Source: CAD feature listing. Evaluate the final solid. Frame: model axes, mm. Coordinates: 2 decimals unless noted, no trailing zeros. Write each loop counter-clockwise with the first axis right and the second up, starting at its lowest first coordinate (ties: lowest second). Pieces come first, ordered by that corner, then holes. Notation, with made-up numbers: M 45,-8 L 77,-8 A32 ccw 77,22 Z; hole C 2,78 d1. An arc over 180 degrees is marked long. Write item = value, one per line. Start each with the question number.
1. Section query A-A (z = -1.8). Output: boundary loops of the cut face in (x, y).
2. Line query: line 1 along Y through (x, z) = (-149, -0.3); line 2 along X through (y, z) = (227, -1.55); line 3 along Y through (x, z) = (-171.5, -0.25). Output: solid intervals per line, ascending.
3. Pull-direction query (X, two-part tool) for faces 1 (the face through (-232.355, 188.231, -1.519)), 2 (the face through (-111.161, 214.644, -1.519)), 3 (the face through (-173, 205, -3)); classes: pulls with the +X half, pulls with the -X half, needs draft (parallel to the pull), parting line crosses it, or undercut.
4. Pin query (flat end, axial travel): pin 1 Ø1.5 at (x, z) = (-133, -2.5) entering from -Y. Return the tip coordinate at first contact, or that it passes through.
```python
from build123d import *

# Parameters (mm, degrees)
SKETCH_1_R      = 9
EXTRUDE_1_DEPTH = 3
FILLET_1_R      = 30
FILLET_2_R      = 0.15


with BuildPart() as part:
    # 草图1 → 凸台-拉伸1 (new body)
    with BuildSketch(Plane.XY):
        with Locations((-244.136401891, 191.197879466)):
            Circle(SKETCH_1_R)
        with Locations((-101.472478495, 222.230200701)):
            Circle(SKETCH_1_R)
        with BuildLine():
            Line((-100.516002841, 217.833024979), (-243.179926237, 186.800703745))
            ThreePointArc((-243.179926237, 186.800703745), (-248.533577612, 190.241403811), (-245.092877546, 195.595055187))
            Line((-245.092877546, 195.595055187), (-102.42895415, 226.627376422))
            ThreePointArc((-102.42895415, 226.627376422), (-97.075302774, 223.186676355), (-100.516002841, 217.833024979))
        make_face()
    extrude(amount=-EXTRUDE_1_DEPTH)

    # 圆角1
    fillet_1_edges = [part.edges().sort_by_distance(p)[0] for p in [
        (-108.132134599, 216.17636055, -1.5),
        (-235.563794478, 188.457368174, -1.5),
        (-237.476745787, 197.251719617, -1.5),
        (-110.045085908, 224.970711992, -1.5),
    ]]
    fillet(fillet_1_edges, radius=FILLET_1_R)

    # 圆角2
    fillet_2_edges = [part.edges().sort_by_distance(p)[0] for p in [
        (-173.760915848, 211.111215804, 0),
        (-173.760915848, 211.111215804, -3),
        (-252.930753333, 189.284928157, 0),
        (-252.930753333, 189.284928157, -3),
        (-171.847964539, 202.316864362, 0),
        (-171.847964539, 202.316864362, -3),
        (-92.678127053, 224.14315201, 0),
        (-92.678127053, 224.14315201, -3),
        (-234.549689719, 198.787190778, 0),
        (-234.549689719, 198.787190778, -3),
        (-232.263398459, 188.276495212, 0),
        (-232.263398459, 188.276495212, -3),
        (-111.059190667, 214.640889389, 0),
        (-111.059190667, 214.640889389, -3),
        (-113.345481927, 225.151584954, 0),
        (-113.345481927, 225.151584954, -3),
    ]]
    fillet(fillet_2_edges, radius=FILLET_2_R)


solid = part.part
```
Results are:
q1.outline = M -241.73,199.87 A9 ccw long -238.34,184.31 A30 cw -225.41,190.67 L -118.29,213.97 A30 cw -103.88,213.56 A9 ccw long -107.27,229.12 A30 cw -120.2,222.76 L -227.32,199.46 A30 cw Z
q2.line_1 = 207.29 to 216.5
q2.line_2 = -110.11 to -93.84
q2.line_3 = 202.39 to 211.6
q3.face_1 = pulls with the +X half
q3.face_2 = undercut
q3.face_3 = needs draft
q4.pin_1 = 210.6
